Here's how the part is built. I have some questions about the finished solid (model axes, mm). Give positions to 0.01 mm unless a question says otherwise; leave off trailing zeros. Write each loop counter-clockwise with the first axis right and the second up, starting at its lowest first coordinate (ties: lowest second). Pieces come first, ordered by that corner, then holes. Notation, with made-up numbers: (74.25, -4) -> (81.25, -4) arc R19 ccw to (81.25, 1) -> close; hole circle Ø2 at (63, 67). An arc over 180 degrees is marked (long way). Put each result on its own line as item: value. Start each with the question number.
from build123d import *

# Parameters (mm, degrees)
SKETCH1_W           = 160
SKETCH1_H           = 150
BOSS_EXTRUDE1_DEPTH = 1
SKETCH3_R           = 1.5
SKETCH3_R_2         = 1.25
SKETCH3_R_3         = 2
SKETCH3_W           = 50
SKETCH3_H           = 4
SKETCH3_W_2         = 3
SKETCH3_H_2         = 14
CUT_EXTRUDE1_DEPTH  = 10


with BuildPart() as part:
    # Sketch1 → Boss-Extrude1 (new body)
    with BuildSketch(Plane.XY):
        Rectangle(SKETCH1_W, SKETCH1_H)
    extrude(amount=BOSS_EXTRUDE1_DEPTH)

    # Sketch3 → Cut-Extrude1 (cut)
    with BuildSketch(Plane.XY.offset(1)):
        with Locations((-77.5, -58)):
            Circle(SKETCH3_R)
        with Locations((77.5, -58)):
            Circle(SKETCH3_R)
        with Locations((77.5, 58)):
            Circle(SKETCH3_R)
        with Locations((-77.5, 58)):
            Circle(SKETCH3_R)
        with Locations((-14.483915959, -11.75)):
            Circle(SKETCH3_R_2)
        with Locations((9.016084041, -11.75)):
            Circle(SKETCH3_R_2)
        with Locations((9.016084041, 11.75)):
            Circle(SKETCH3_R_2)
        with Locations((-14.483915959, 11.75)):
            Circle(SKETCH3_R_2)
        with Locations((-41.40147673, 0)):
            Circle(SKETCH3_R_3)
        with Locations((-41.40147673, -21.215676989)):
            Circle(SKETCH3_R_3)
        with Locations((-41.40147673, 21.215676989)):
            Circle(SKETCH3_R_3)
        with Locations((-41.40147673, -42.218866747)):
            Circle(SKETCH3_R_3)
        with Locations((-41.40147673, 42.218866747)):
            Circle(SKETCH3_R_3)
        with Locations((55, 73)):
            Rectangle(SKETCH3_W, SKETCH3_H)
        with Locations((-14.483915959, 0)):
            Rectangle(SKETCH3_W_2, SKETCH3_H_2)
    extrude(amount=-CUT_EXTRUDE1_DEPTH, mode=Mode.SUBTRACT)


solid = part.part
1) I want a section at A-A, the plane y = 0. Write out the boundary of the cut face in (x, z).
2) I need wall thicknesses on probe 1 along Y at (x, z) = (-15.5, 0.65); probe 2 along X at (y, z) = (6.5, 0.4); probe 3 along Y at (x, z) = (49, 0.65). Which ranges of each line are inside material? Lowest first, please.
3) I'm going to push flat-ended pins straight in: pin 1 Ø3.5 at (x, y) = (-77.5, -58) entering from -Z; pin 2 Ø0.5 at (y, z) = (72.5, 0.5) entering from +X. Where does each tip first touch, or does it pass through?
4) Thinking about a two-plate mould opening in Y: for faces 1 (the flat face through (-1, 1, 1)), 2 (the cylindrical face through (-43.4, 0.1, 0.5)), which applies, released by +Y, released by -Y, zero draft, split by the parting line, or undercut?
5) I want a section at B-B, the plane x = 67. Write out the boundary of the cut face in (y, z).
Established:
1. outline: (-80, 0) -> (-43.4, 0) -> (-43.4, 1) -> (-80, 1) -> close; (-39.4, 0) -> (-15.98, 0) -> (-15.98, 1) -> (-39.4, 1) -> close; (-12.98, 0) -> (80, 0) -> (80, 1) -> (-12.98, 1) -> close
2. probe 1: y = -75 to -12.48, -11.02 to -7, 7 to 11.02, 12.48 to 75
2. probe 2: x = -80 to -15.98, -12.98 to 80
2. probe 3: y = -75 to 71
3. pin 1: stops at z = 0
3. pin 2: stops at x = 30
4. face 1: zero draft
4. face 2: undercut
5. outline: (-75, 0) -> (71, 0) -> (71, 1) -> (-75, 1) -> close
